For this review, use the dimensioned drawing (mm, ordinates from the lowest corner) and the shaded views. A direction names the side the tool comes from. Coordinates: 2 decimals unless noted, no trailing zeros. Write each loop counter-clockwise with the first axis right and the second up, starting at its lowest first coordinate (ties: lowest second). Pieces come first, ordered by that corner, then holes. Notation, with made-up numbers: M 89,29 L 143,29 A26 ccw 143,59 Z; hole C -24,3 d3. An arc over 180 degrees is marked long. One line per question, with ' | ' between items.
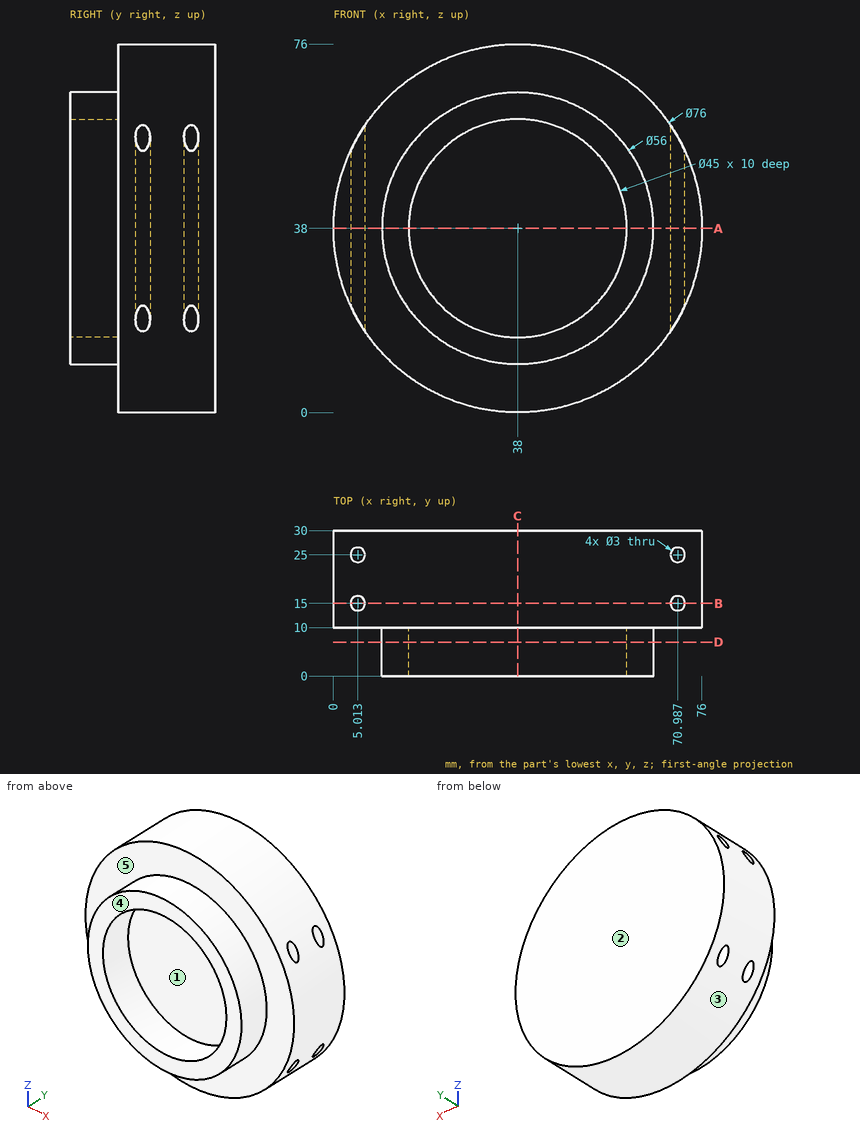
1) The part is to be moulded in two halves that separate along X. For the marked faces 1, 2 and 3, say which applies: +X half, -X half, draft (parallel to the pull), parting line (faces both ways), or undercut.
Responses:
face 1: undercut | face 2: draft | face 3: parting line
2) We need section B-B on y = 15. State the section outline as (x, z) points, then the cut area to 3 significant figures.
Responses:
outline: M 3.51,22.04 L 3.51,53.96 A38 ccw Z; M 6.51,16.73 A38 ccw 69.49,16.73 L 69.49,59.27 A38 ccw 6.51,59.27 Z; M 72.49,22.04 A38 ccw 72.49,53.96 Z | area: 4,310 mm^2
3) Insertion check: pin 1 Ø1.5 at (x, y) = (31, 19.5) entering from -Z; pin 2 Ø2 at (y, z) = (18, 27.5) entering from +X; pin 3 Ø2 at (x, y) = (62, 6) entering from +Z; pin 4 Ø2.5 at (x, y) = (5.01, 25) entering from -Z. Each pin has a flat end and moves straight along its axis. Give the tip position at first contact, or say it passes through.
Responses:
pin 1: z = 0.52 | pin 2: x = 74.79 | pin 3: z = 53.97 | pin 4: through
4) To check wall thickness, follow line 1 along X through (y, z) = (25, 31); line 2 along X through (y, z) = (25, 40.5); line 3 along Z through (x, y) = (53.5, 2). State the ranges of each line that lie inside material, in increasing order. Write a range as [from, to].
Responses:
line 1: [0.65, 3.51], [6.51, 69.49], [72.49, 75.35] | line 2: [0.08, 3.51], [6.51, 69.49], [72.49, 75.92] | line 3: [14.68, 21.69], [54.31, 61.32]
5) Machinability: for the marked faces 4 and 5, which of the approach directions +Z, -Z, +X, -X, +Y, -Y give a long, thin tool a straight path to every point of the face, cutting with its end or side? Answer none if there is none.
Responses:
face 4: +Z, -Z, +X, -X, -Y | face 5: -Y
6) We need section D-D on y = 7. State the section outline as (x, z) points.
Responses:
outline: C 38,38 d56; hole C 38,38 d45
7) We need section A-A on z = 38. State the section outline as (x, y) points.
Responses:
outline: M 0,10 L 10,10 L 10,0 L 15.5,0 L 15.5,10 L 60.5,10 L 60.5,0 L 66,0 L 66,10 L 76,10 L 76,30 L 0,30 Z; hole C 5.01,15 d3; hole C 5.01,25 d3; hole C 70.99,15 d3; hole C 70.99,25 d3
8) We need section C-C on x = 38. State the section outline as (y, z) points.
Responses:
outline: M 0,10 L 10,10 L 10,0 L 30,0 L 30,76 L 10,76 L 10,66 L 0,66 L 0,60.5 L 10,60.5 L 10,15.5 L 0,15.5 Z
